Check sheet for the modelled part. Datum: model origin and axes. Units: mm. A direction names the side the tool comes from. Coordinates: 2 decimals unless noted, no trailing zeros. Write each loop counter-clockwise with the first axis right and the second up, starting at its lowest first coordinate (ties: lowest second). Pieces come first, ordered by that corner, then holes. Notation, with made-up numbers: (28, -33) - (80, -33) arc R12 ccw to (80, -26) - close; hole circle Ø3 at (-7, -32). An arc over 180 degrees is marked (long way). Write each question's results on one line, items separated by ' | '.
from build123d import *

# Parameters (mm, degrees)
ESBO_O1_W                  = 125
ESBO_O1_H                  = 50
RESSALTO_EXTRUS_O1_DEPTH   = 2.5
ESBO_O2_R                  = 1.6
CORTE_EXTRUS_O2_DEPTH      = 2.5
CORTE_EXTRUS_O3_DEPTH      = 1.5
CORTE_EXTRUS_O5_DEPTH      = 113.726994752
CORTE_EXTRUS_O5_DEPTH_BACK = 113.726994752
ESBO_O12_R                 = 2.75
CORTE_EXTRUS_O6_DEPTH      = 2
ESBO_O19_R                 = 1.5
CORTE_EXTRUS_O7_DEPTH      = 2
FILETE1_R                  = 2


with BuildPart() as part:
    # Esboço1 → Ressalto-extrusão1 (new body)
    with BuildSketch(Plane.XY):
        with Locations((44.657564369, 9.905325444)):
            Rectangle(ESBO_O1_W, ESBO_O1_H)
    extrude(amount=RESSALTO_EXTRUS_O1_DEPTH)

    # Esboço2 → Corte-extrusão2 (cut)
    with BuildSketch(Plane.XY.offset(2.5)):
        with Locations((34.157564369, 22.905325444)):
            Circle(ESBO_O2_R)
        with Locations(Location((34.157564369, -3.094674556, 0), (0, 0, 180))):
            Circle(ESBO_O2_R)
        with Locations((52.157564369, -3.094674556)):
            Circle(ESBO_O2_R)
        with Locations(Location((52.157564369, 22.905325444, 0), (0, 0, 180))):
            Circle(ESBO_O2_R)
    extrude(amount=-CORTE_EXTRUS_O2_DEPTH, mode=Mode.SUBTRACT)

    # Esboço3 → Corte-extrusão3 (cut)
    with BuildSketch(Plane.XY.offset(2.5)):
        Polygon((-17.842435631, 32.905325444), (-17.842435631, 9.905325444), (-15.842435631, 9.905325444), (-15.842435631, 32.905325444), (107.157564369, 32.905325444), (107.157564369, 34.905325444), (-15.842435631, 34.905325444), (-17.842435631, 34.905325444), align=None)
        Polygon((-15.842435631, 9.905325444), (-17.842435631, 9.905325444), (-17.842435631, -13.094674556), (-17.842435631, -15.094674556), (-15.842435631, -15.094674556), (107.157564369, -15.094674556), (107.157564369, -13.094674556), (-15.842435631, -13.094674556), align=None)
    extrude(amount=-CORTE_EXTRUS_O3_DEPTH, mode=Mode.SUBTRACT)

    # Esboço4 → Corte-extrusão5 (cut, two sides: drawn at the far end of the back side and taken through both)
    with BuildSketch(Plane.XY.offset(2.5).offset(-CORTE_EXTRUS_O5_DEPTH_BACK)):
        Polygon((0.690585312, 9.905325444), (10.419553485, -10.094674556), (18.419553485, -10.094674556), (8.690585312, 9.905325444), (18.419553485, 29.905325444), (10.419553485, 29.905325444), align=None)
        Polygon((20.690585312, 9.905325444), (30.419553485, 29.905325444), (22.419553485, 29.905325444), (12.690585312, 9.905325444), (22.419553485, -10.094674556), (30.419553485, -10.094674556), align=None)
        Polygon((30.419553485, 23.738176067), (23.690585312, 9.905325444), (30.419553485, -3.927525179), align=None)
        Polygon((-11.309414688, 9.905325444), (-1.580446515, -10.094674556), (6.419553485, -10.094674556), (-3.309414688, 9.905325444), (6.419553485, 29.905325444), (-1.580446515, 29.905325444), align=None)
        Polygon((95.624543426, 9.905325444), (85.895575254, 29.905325444), (77.895575254, 29.905325444), (87.624543426, 9.905325444), (77.895575254, -10.094674556), (85.895575254, -10.094674556), align=None)
        Polygon((83.624543426, 9.905325444), (73.895575254, 29.905325444), (65.895575254, 29.905325444), (75.624543426, 9.905325444), (65.895575254, -10.094674556), (73.895575254, -10.094674556), align=None)
        Polygon((71.624543426, 9.905325444), (61.895575254, 29.905325444), (53.895575254, 29.905325444), (63.624543426, 9.905325444), (53.895575254, -10.094674556), (61.895575254, -10.094674556), align=None)
        Polygon((60.624543426, 9.905325444), (53.895575254, -3.927525179), (53.895575254, 23.738176067), align=None)
    extrude(amount=CORTE_EXTRUS_O5_DEPTH + CORTE_EXTRUS_O5_DEPTH_BACK, mode=Mode.SUBTRACT)

    # Esboço12 → Corte-extrusão6 (cut)
    with BuildSketch(Plane.XY.offset(2.5)):
        with Locations((97.607564369, 24.905325444)):
            Circle(ESBO_O12_R)
        with Locations((97.607564369, -5.094674556)):
            Circle(ESBO_O12_R)
    extrude(amount=-CORTE_EXTRUS_O6_DEPTH, mode=Mode.SUBTRACT)

    # Esboço19 → Corte-extrusão7 (cut)
    with BuildSketch(Plane.XY.offset(0.5)):
        with Locations((97.607564369, 24.905325444)):
            Circle(ESBO_O19_R)
        with Locations((97.607564369, -5.094674556)):
            Circle(ESBO_O19_R)
    extrude(amount=-CORTE_EXTRUS_O7_DEPTH, mode=Mode.SUBTRACT)

    # Filete1
    filete1_edges = [part.edges().sort_by_distance(p)[0] for p in [
        (-17.842435631, -15.094674556, 0.5),
        (-15.842435631, -13.094674556, 1.75),
        (-17.842435631, 34.905325444, 0.5),
        (-15.842435631, 32.905325444, 1.75),
        (107.157564369, -15.094674556, 0.5),
        (107.157564369, -13.094674556, 1.75),
        (107.157564369, 32.905325444, 1.75),
        (107.157564369, 34.905325444, 0.5),
    ]]
    fillet(filete1_edges, radius=FILETE1_R - 0.0001)  # a hair under: the kernel refuses the full size


solid = part.part
1. Material ranges on L1, parallel to Y at x = 14, z = 1.3; L2, parallel to Y at x = 58, z = 2.2; L3, parallel to Y at x = 63, z = 0.45, recorded low to high. Write a range as [from, to].
Values follow:
L1: y = [-13.09, -10.09], [-1.01, 7.21], [12.6, 20.82], [29.91, 32.91] | L2: y = [-13.09, -10.09], [-1.66, 4.51], [15.3, 21.47], [29.91, 32.91] | L3: y = [-15.09, -7.82], [8.62, 11.19], [27.63, 34.91]
2. Sectioned sample at A-A (x = 40.5). Record the cut outline in (y, z), then the cut area to 3 significant figures.
Values follow:
outline: (-15.09, 0) - (34.91, 0) - (34.91, 1) - (32.91, 1) - (32.91, 2.5) - (-13.09, 2.5) - (-13.09, 1) - (-15.09, 1) - close | area: 119 mm^2
3. Access from +Z, -Z, +X, -X, +Y, -Y to the whole of each face (thin tool, end or side, straight path). Record for faces 1 (the flat face through (70, -10.095, 1)), 2 (the cylindrical face through (97.25, -2.37, 1.51)), 3 (the flat face through (45, 10, 2.5)).
Values follow:
face 1: +Z, -Z | face 2: +Z | face 3: +Z, +X, -X, +Y, -Y
4. Go/stop test with flat-tipped pins: pin 1 (1.2 mm diameter, centred on x = 38, z = 2, fed in from -Y); pin 2 (3 mm diameter, centred on x = 97, y = -5.5, fed in from +Z); pin 3 (0.8 mm diameter, centred on y = 16.5, z = 2, fed in from -X). Record where each tip stops, or that it passes through.
Values follow:
pin 1: stops at y = -13.09 | pin 2: stops at z = 0.5 | pin 3: stops at x = -15.84
5. Sectioned sample at C-C (x = -5). Record the cut outline in (y, z), then the cut area to 3 significant figures.
Values follow:
outline: (-15.09, 0) - (-3.07, 0) - (-3.07, 2.5) - (-13.09, 2.5) - (-13.09, 1) - (-15.09, 1) - close; (22.88, 0) - (34.91, 0) - (34.91, 1) - (32.91, 1) - (32.91, 2.5) - (22.88, 2.5) - close | area: 54.1 mm^2
6. Draft check along X on faces 4 (the flat face through (25.62, -0.23, 1.23)), 5 (the flat face through (44, -14, 1)), 6 (the flat face through (58.69, 20.05, 1.23)). Enter one of: pulls with the +X half, pulls with the -X half, needs draft (parallel to the pull), parting line crosses it, or undercut.
Values follow:
face 4: undercut | face 5: needs draft | face 6: undercut
7. Sectioned sample at B-B (x = 56.5). Record the cut outline in (y, z).
Values follow:
outline: (-15.09, 0) - (-10.09, 0) - (-10.09, 2.5) - (-13.09, 2.5) - (-13.09, 1) - (-15.09, 1) - close; (-4.74, 0) - (1.43, 0) - (1.43, 2.5) - (-4.74, 2.5) - close; (18.38, 0) - (24.55, 0) - (24.55, 2.5) - (18.38, 2.5) - close; (29.91, 0) - (34.91, 0) - (34.91, 1) - (32.91, 1) - (32.91, 2.5) - (29.91, 2.5) - close
8. Sectioned sample at D-D (z = 1.4). Give the number of separate pieces and of enclosed holes in the cut face, then the cut area to 3 significant figures.
Values follow:
separate pieces: 1 | enclosed holes: 14 | area: 3,470 mm^2
